Geometry: final body of the model. Coordinates: model frame, mm. Give positions to 0.01 mm unless a question says otherwise; leave off trailing zeros. Loops run counter-clockwise (first coordinate to the right, second up) from the corner with the lowest first, then second, coordinate; pieces in that order, holes last.
from build123d import *

# Parameters (mm, degrees)
F0_W     = 60
F0_H     = 16
F0_R     = 6.95
F1_DEPTH = 1.5


# Not quite as in the source:
# - a fillet or chamfer that OpenCascade refuses, or shapes differently, is made with other operations: its cross-section is extruded or revolved along the edge and cut away or added


with BuildPart() as f1:
    # F0 (on Top) → F1 (new body)
    with BuildSketch(Plane.XY):
        Rectangle(F0_W, F0_H)
        Circle(F0_R, mode=Mode.SUBTRACT)
    extrude(amount=F1_DEPTH)

    # F2: chamfer of 1.5 on 1 edges, made by hand

    # F2_s1 → F2_t2 (revolve, cut)
    with BuildSketch(Plane.XZ):
        Polygon((6.95, 1.5), (8.45, 0), (6.95, 0), align=None)
    revolve(axis=Axis((0, 0, 0), (0, 0, 1)), mode=Mode.SUBTRACT)


solid = f1.part
Item 1: Section query C-C on z = 0.8. Return loops of the section in (x, y), plus the area to 3 significant figures.
Values follow:
outline: (-30, -8) - (30, -8) - (30, 8) - (-30, 8) - close; hole circle Ø15.3 at (0, 0)
area: 776 mm2
Item 2: Section query A-A on y = 0. Return loops of the section in (x, z).
Values follow:
outline: (-30, 0) - (-8.45, 0) - (-6.95, 1.5) - (-30, 1.5) - close; (6.95, 1.5) - (8.45, 0) - (30, 0) - (30, 1.5) - close
Item 3: Pin query (flat end, axial travel): pin 1 (5 mm diameter, centred on x = 18, y = 1.5, fed in from -Z). Return the tip coordinate at first contact, or that it passes through.
Values follow:
pin 1: stops at z = 0
Item 4: Ray query, probe 1 along X at (y, z) = (3, 0.1); probe 2 along Y at (x, z) = (-5.5, 1.05); probe 3 along X at (y, z) = (6.25, 1.15). Return the intervals inside material, ascending.
Values follow:
probe 1: x = -30 to -7.79, 7.79 to 30
probe 2: y = -8 to -4.95, 4.95 to 8
probe 3: x = -30 to -3.77, 3.77 to 30
Item 5: Section query B-B on x = 0. Return loops of the section in (y, z).
Values follow:
outline: (-8, 0.45) - (-6.95, 1.5) - (-8, 1.5) - close; (6.95, 1.5) - (8, 0.45) - (8, 1.5) - close
